Verification items for this drawing (mm, ordinates from the low corner). A direction names the side the tool comes from. Round coordinates to 2 decimals unless told otherwise and drop trailing zeros. Loops run counter-clockwise (first coordinate to the right, second up) from the corner with the lowest first, then second, coordinate; pieces in that order, holes last. Notation, with made-up numbers: M 84,12.25 L 120,12.25 A24 cw 120,50.25 Z; hole C -2,-1 d2. An arc over 180 degrees is marked long. One line per item, written item: value.
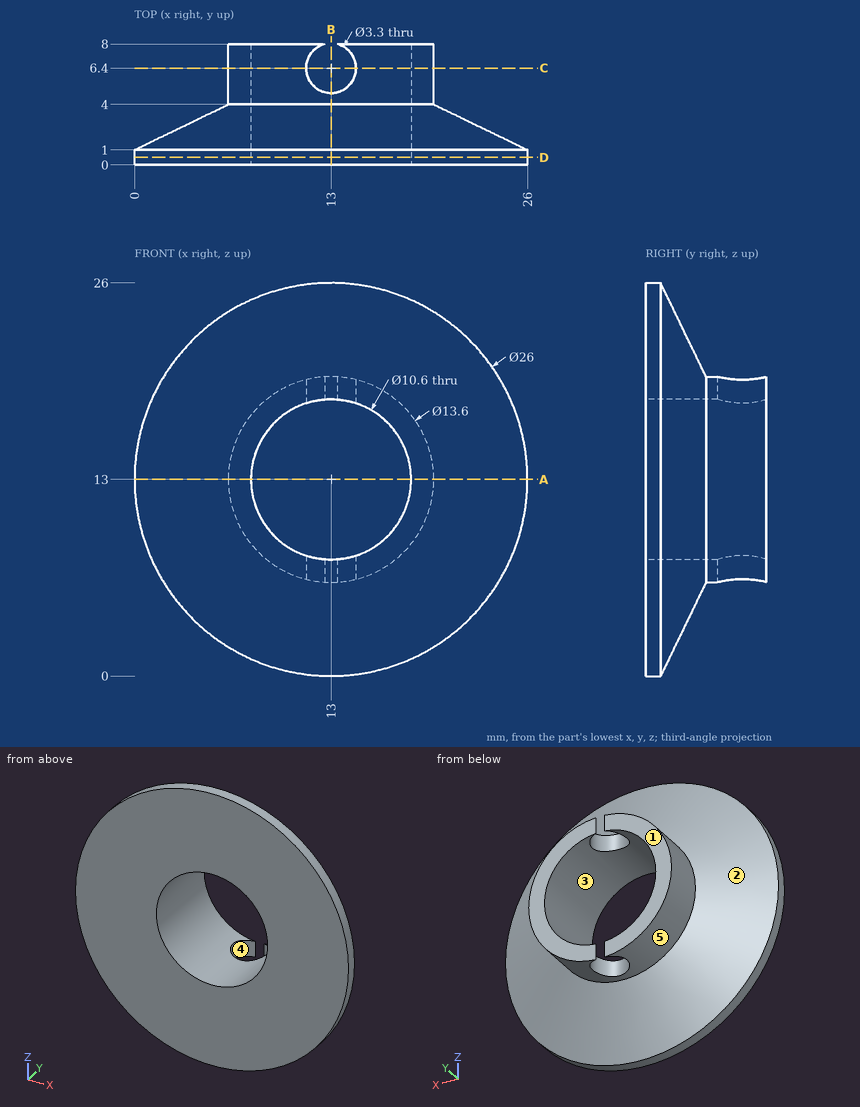
(1) Depth check by flat-ended pin: pin 1 Ø3 at (x, y) = (13, 6.4) entering from +Z; pin 2 Ø3 at (x, y) = (15.5, 2) entering from -Z. Enter the tip coordinate at first touch or a pass-through.
Completed:
pin 1: passes through
pin 2: stops at z = 0.07
(2) Sectioned sample at D-D on y = 0.5. Enter the section's corners in (x, z), and give its area (3 significant figures).
Completed:
outline: C 13,13 d26; hole C 13,13 d10.6
area: 443 mm^2
(3) Sectioned sample at C-C on y = 6.4. Enter the section's corners in (x, z).
Completed:
outline: M 11.35,6.4 L 11.35,7.96 A5.3 cw 11.35,18.04 L 11.35,19.6 A6.8 ccw Z; M 14.65,6.4 A6.8 ccw 14.65,19.6 L 14.65,18.04 A5.3 cw 14.65,7.96 Z
(4) Tool access check on the marked faces 4 and 5. Record the directions out of +Z, -Z, +X, -X, +Y, -Y that give a thin tool (end or side, any length) a straight path to the whole face; none if there is none.
Completed:
face 4: +Z, -Z
face 5: +Y
(5) Sectioned sample at A-A on z = 13. Enter the section's corners in (x, y), and give its area (3 significant figures).
Completed:
outline: M 0,0 L 7.7,0 L 7.7,8 L 6.2,8 L 6.2,4 L 0,1 Z; M 18.3,0 L 26,0 L 26,1 L 19.8,4 L 19.8,8 L 18.3,8 Z
area: 55.0 mm^2
(6) Sectioned sample at B-B on x = 13. Enter the section's corners in (y, z).
Completed:
outline: M 0,0 L 1,0 L 4,6.2 L 4.75,6.2 L 4.75,7.7 L 0,7.7 Z; M 0,18.3 L 4.75,18.3 L 4.75,19.8 L 4,19.8 L 1,26 L 0,26 Z
(7) Thickness scan on L1, parallel to Y at x = 13, z = 7.45; L2, parallel to X at y = 6.75, z = 14.5; L3, parallel to X at y = 7.75, z = 9.25. Record the ranges inside material, lowest first. Write a range as from..to.
Completed:
L1: y = 0..4.75
L2: x = 6.37..7.92, 18.08..19.63
L3: x = 7.33..9.25, 16.75..18.67
(8) Mould release check, pull along Z, two halves, no side actions. Record for the marked faces 1, 2 and 3: +Z half, -Z half, draft (parallel to the pull), parting line (faces both ways), or undercut.
Completed:
face 1: draft
face 2: parting line
face 3: undercut
